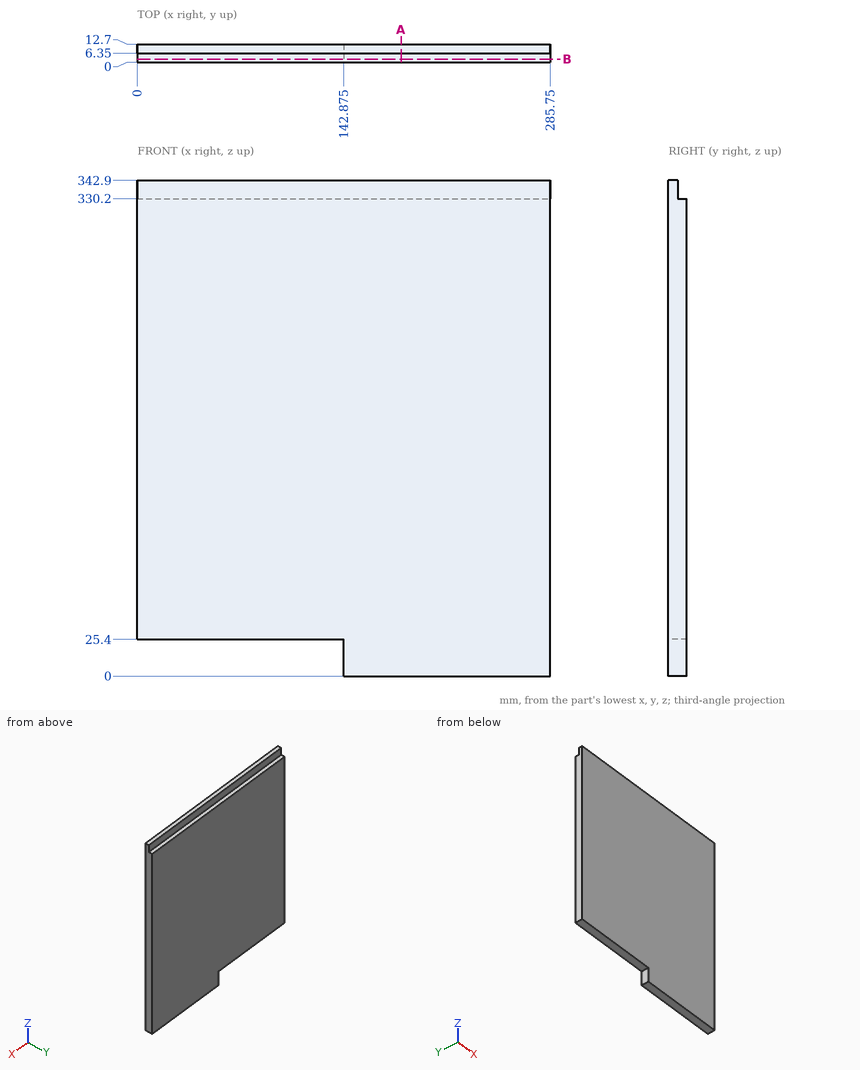
Check sheet for the drawn part. Datum: minimum x, y, z corner. Units: mm. Round coordinates to 2 decimals unless told otherwise and drop trailing zeros. Loops run counter-clockwise (first coordinate to the right, second up) from the corner with the lowest first, then second, coordinate; pieces in that order, holes last. Notation, with made-up numbers: (88, -33) - (97, -33) arc R23 cw to (97, -2) - close; hole circle Ø5 at (-19.5, -7.75). An arc over 180 degrees is marked (long way). Write each question's results on one line, items separated by ' | '. Start each with the question number.
Q1. Gauge pin test, flat ends, axial feed: P1, Ø2, axis at x = 61.5, y = 9, coming from the -Z side; P2, Ø7, axis at x = 98.5, y = 10.5, coming from the +Z side; P3, Ø4, axis at y = 5.5, z = 15.5, coming from the -X side (3 decimals). Record the tip position at first contact, or that the pin passes through.
Q2. Cross-section at A-A on x = 182.5. Enter the section's corners in (y, z).
Q3. Thickness scan on line 1 (Z direction, x = 112, y = 11.5); line 2 (Z direction, x = 238, y = 9.75); line 3 (X direction, y = 1.5, z = 14) (3 decimals). Record the ranges inside material, lowest first. Write a range as [from, to].
Q4. Cross-section at B-B on y = 2.25. Enter the section's corners in (x, z) (3 decimals), and give its area (3 significant figures).
Answers below:
1) P1: stops at z = 25.4 | P2: stops at z = 330.2 | P3: stops at x = 142.875
2) outline: (0, 0) - (12.7, 0) - (12.7, 330.2) - (6.35, 330.2) - (6.35, 342.9) - (0, 342.9) - close
3) line 1: z = [25.4, 330.2] | line 2: z = [0, 330.2] | line 3: x = [142.875, 285.75]
4) outline: (0, 25.4) - (142.875, 25.4) - (142.875, 0) - (285.75, 0) - (285.75, 342.9) - (0, 342.9) - close | area: 94,400 mm²
